Input: part model. Units: mm. Frame: model coordinates. A direction names the side the tool comes from. Round coordinates to 2 decimals unless told otherwise and drop trailing zeros. Loops run counter-clockwise (first coordinate to the right, second up) from the corner with the lowest first, then second, coordinate; pieces in that order, holes last. Notation, with made-up numbers: (28.5, 30.25) - (42.5, 30.25) arc R12 cw to (42.5, 34.25) - close; hole circle Ø3 at (7, 45). An arc over 180 degrees is marked (long way). Write each question's results on one line, items separated by ' | '.
Autodesk Inventor part; units mm, degrees
ref_plane "YZ Plane" through (0, 0, 0) normal (1, 0, 0) x (0, 1, 0)
ref_plane "XZ Plane" through (0, 0, 0) normal (0, 1, 0) x (-1, 0, 0)
ref_plane "XY Plane" through (0, 0, 0) normal (0, 0, 1) x (1, 0, 0)
sketch "Sketch1" plane through (0, 0, 0) normal (0, 1, 0) x (-1, 0, 0)
  line L0 (5, 0) -> (31, 0)
  line L1 (36, -30) -> (36, -120)
  line L2 (31, -150) -> (5, -150)
  line L3 (0, -120) -> (0, -30)
  circle A0 centre (18, -25) radius 5.1
  circle A1 centre (18, -55) radius 5.1
  circle A2 centre (18, -85) radius 5.1
  circle A3 centre (18, -125) radius 5.1
  line L4 (36, -30) -> (31, -30)
  line L5 (31, -30) -> (31, -40)
  line L6 (31, -40) -> (36, -40)
  line L7 (36, -120) -> (31, -120)
  line L8 (31, -120) -> (31, -110)
  line L9 (31, -110) -> (36, -110)
  line L10 (0, -30) -> (5, -30)
  line L11 (5, -30) -> (5, -40)
  line L12 (5, -40) -> (0, -40)
  line L13 (0, -120) -> (5, -120)
  line L14 (5, -120) -> (5, -110)
  line L15 (0, -110) -> (5, -110)
  circle A4 centre (18, -25) radius 2.25
  circle A5 centre (18, -55) radius 2.25
  circle A6 centre (18, -85) radius 2.25
  circle A7 centre (18, -125) radius 2.25
  line L16 (5, 0) -> (0, -30)
  line L17 (31, -150) -> (36, -120)
  line L18 (5, -150) -> (0, -120)
  line L19 (31, 0) -> (36, -30)
  line L20 (18, -100) -> (13, -105)
  line L21 (13, -105) -> (18, -110)
  line L22 (23, -105) -> (18, -110)
  line L23 (23, -105) -> (18, -100)
  line L24 (21, -114.95) -> (18, -117.95)
  line L25 (15, -114.95) -> (18, -117.95)
  line L26 (15, -114.95) -> (18, -111.95)
  line L27 (18, -111.95) -> (21, -114.95)
  line L28 (21, -95.05) -> (18, -98.05)
  line L29 (18, -98.05) -> (15, -95.05)
  line L30 (15, -95.05) -> (18, -92.05)
  line L31 (18, -92.05) -> (21, -95.05)
  line L32 (31, -150) -> (28, -150)
  line L33 (5, -150) -> (8, -150)
  line L34 (8, -148) -> (28, -148)
  line L35 (8, -148) -> (8, -144)
  line L36 (8, -144) -> (28, -144)
  line L37 (28, -144) -> (28, -148)
  line L38 (31, 0) -> (28, 0)
  line L39 (5, 0) -> (8, 0)
  line L40 (8, -2) -> (28, -2)
  line L41 (28, -2) -> (28, -6)
  line L42 (28, -6) -> (8, -6)
  line L43 (8, -6) -> (8, -2)
  line L44 (36, -75) -> (36, -83)
  line L45 (36, -75) -> (36, -67)
  line L46 (36, -67) -> (28, -75)
  line L47 (36, -83) -> (28, -75)
  line L48 (0, -75) -> (0, -83)
  line L49 (0, -75) -> (0, -67)
  line L50 (0, -67) -> (8, -75)
  line L51 (0, -83) -> (8, -75)
  point P0 (0, 0)
  point P1 (18, 0)
  point P2 (18, -150)
  dimension "d2" = 10.2
  dimension "d3" = 25
  dimension "d4" = 10.2
  dimension "d5" = 30
  dimension "d6" = 10.2
  dimension "d7" = 30
  dimension "d8" = 10.2
  dimension "d9" = 40
  dimension "d10" = 25
  dimension "d12" = 5
  dimension "d13" = 10
  dimension "d15" = 10
  dimension "d17" = 5
  dimension "d19" = 5
  dimension "d22" = 4.5
  dimension "d23" = 4.5
  dimension "d24" = 4.5
  dimension "d25" = 4.5
  dimension "d38" = 3
  dimension "d39" = 2
  dimension "d41" = 2
  dimension "d42" = 4
  dimension "d44" = 2
  dimension "d45" = 3
  dimension "d46" = 4
  dimension "d50" = 8
  dimension "d51" = 8
extrude "Extrusion1" add sketch "Sketch1" along normal blind 5 contours L0 L19 L4 L5 L6 L1 L46 L47 L9 L8 L7 L17 L2 L18 L13 L14 L15 L3 L51 L50 L12 L11 L10 L16
extrude "Extrusion2" add sketch "Sketch1" along normal blind 1 contours A0 | A1 | A2 | A3
sketch "Sketch2" plane through (0, 5, 0) normal (0, 1, 0) x (1, 0, 0)
  line L0 (-36, 120) -> (-31, 120)
  line L1 (-33.5, 120) -> (-33.5, 135)
  line L2 (-31, 150) -> (-36, 120)
  line L3 (-33.5, 120) -> (-35.9995, 120)
  line L4 (-35.9995, 120) -> (-33.5, 135)
  line L5 (-31, 30) -> (-36, 30)
  line L6 (-33.5, 30) -> (-33.5, 15)
  line L7 (-36, 30) -> (-31, 0)
  line L8 (-33.5, 15) -> (-36, 30)
  line L9 (-36, 30) -> (-33.5, 30)
  point P0 (0, 0)
  dimension "d52" = 15
extrude "Extrusion3" add sketch "Sketch2" along normal blind 20
sketch "Sketch3" plane through (-36, 0, -120) normal (0, 0, 1) x (1, 0, 0)
  line L0 (2.5, 5) -> (2.5, 25)
  line L1 (0, 0) -> (0, 5)
  line L2 (2.5, 25) -> (0, 25)
  line L3 (0, 25) -> (0, 5)
  line L4 (0, 5) -> (2.5, 5)
  line L5 (2.5, 5) -> (2.5, 25)
  point P0 (36, 0)
extrude "Extrusion4" add sketch "Sketch3" along normal blind 20
sketch "Sketch4" plane through (-31, 0, -30) normal (0, 0, -1) x (-1, 0, 0)
  line L0 (5, 0) -> (5, 25)
  line L1 (2.5, 5) -> (5, 5)
  line L2 (5, 5) -> (5, 25)
  line L3 (5, 25) -> (2.5, 25)
  line L4 (2.5, 25) -> (2.5, 5)
  point P0 (-31, 0)
extrude "Extrusion5" add sketch "Sketch4" along normal blind 20
sketch "Sketch5" plane through (-33.5, 5, -135) normal (1, 0, 0) x (0, 0, -1)
  line L0 (0, 20) -> (-35, 20)
  line L1 (0, 20) -> (0, 10)
  line L2 (0, 0) -> (0, 20)
  line L3 (-35, 0) -> (-35, 20)
  line L4 (-35, 10) -> (-35, 20)
  line L5 (-35, 20) -> (0, 20)
  line L6 (-85, 20) -> (-85, 0)
  line L7 (-120, 20) -> (-85, 20)
  line L8 (-85, 10) -> (-120, 10)
  line L9 (-120, 10) -> (-120, 20)
  line L10 (-120, 20) -> (-85, 20)
  line L11 (-85, 20) -> (-85, 10)
  line L12 (0, 10) -> (-35, 10)
  line L13 (-35, 10) -> (-35, 20)
  line L14 (-35, 20) -> (0, 20)
  line L15 (0, 20) -> (0, 10)
  line L16 (0, 0) -> (-35, 0)
  line L17 (-35, 0) -> (-35, 15)
  line L18 (-35, 15) -> (0, 15)
  line L19 (0, 15) -> (0, 0)
  line L20 (-35, 15) -> (0, 15)
  line L21 (0, 15) -> (0, 20)
  line L22 (0, 20) -> (-35, 20)
  line L23 (-35, 20) -> (-35, 15)
  line L24 (-85, 15) -> (-120, 15)
  line L25 (-120, 15) -> (-120, 20)
  line L26 (-120, 20) -> (-85, 20)
  line L27 (-85, 20) -> (-85, 15)
  point P0 (-135, -5)
extrude "Extrusion6" add sketch "Sketch5" along normal blind 20 contours L1 L18 L3 L0 | L6 L24 L9 L7
fillet "Fillet1" radius 2 4 edges at (-13.5, 25, -117.5) (-13.5, 25, -32.5) (-23.5, 25, -15) (-23.5, 25, -135)
sketch "Sketch6" plane through (0, 25, 0) normal (0, 1, 0) x (1, 0, 0)
  circle A0 centre (-18, 125) radius 2.25
  circle A1 centre (-18, 125) radius 2.25
  circle A2 centre (-18, 25) radius 2.25
  circle A3 centre (-18, 25) radius 2.25
  circle A4 centre (-18, 125) radius 2.5
  circle A5 centre (-18, 25) radius 2.5
  point P0 (0, 0)
  dimension "d62" = 5
  dimension "d63" = 5
extrude "Extrusion7" cut sketch "Sketch6" against normal blind 20 contours A0 | A2 | A4 | A5
properties part number "SideV1"
1. Section query D-D, the plane z = -102. Output: boundary loops of the cut face in (x, y), plus the area to 3 significant figures.
Answer:
outline: (-36, 0) - (-20, 0) - (-20, 5) - (-33.5, 5) - (-33.5, 20) - (-13.5, 20) - (-13.5, 23) arc R2 ccw to (-15.5, 25) - (-36, 25) - close; (-16, 0) - (0, 0) - (0, 5) - (-16, 5) - close | area: 309 mm^2
2. Contact query for flat-ended pins moving along their axis: pin 1 (1.5 mm diameter, centred on x = -19, y = 21.5, fed in from -Z); pin 2 (5.5 mm diameter, centred on y = 1.5, z = -116, fed in from +X); pin 3 (12 mm diameter, centred on y = 12.5, z = -18.5, fed in from -X). Output: stop coordinate, or through.
Answer:
pin 1: z = -135 | pin 2: x = -5 | pin 3: x = -35.08
3. Section query A-A, the plane y = 21.5. Output: boundary loops of the cut face in (x, z), plus the area to 3 significant figures.
Answer:
outline: (-36, -120) - (-33.5, -135) - (-13.5, -135) - (-13.5, -100) - (-36, -100) - close; (-36, -50) - (-13.5, -50) - (-13.5, -15) - (-33.5, -15) - (-36, -30) - close; hole circle Ø5 at (-18, -125); hole circle Ø5 at (-18, -25) | area: 1,500 mm^2
4. Set-up query: faces 1 (the flat face through (-16.48, 2.46, -93.57)), 2 (the cylindrical face through (-18.33, 22.54, -127.48)), 3 (the flat face through (-34, 2, -30)), 4 (the flat face through (-27.2, 20.2, -50)). Return all of +Z, -Z, +X, -X, +Y, -Y with unobstructed straight access to the full face (end or side cutting, diameter ignored); none if empty.
Answer:
face 1: +Y, -Y | face 2: +Y | face 3: -X, -Y | face 4: +X, -X, +Y
5. Section query C-C, the plane y = 6.75. Output: boundary loops of the cut face in (x, z), plus the area to 4 significant figures.
Answer:
outline: (-36, -120) - (-33.5, -135) - (-33.5, -100) - (-36, -100) - close; (-36, -50) - (-33.5, -50) - (-33.5, -15) - (-36, -30) - close | area: 137.5 mm^2
6. Section query B-B, the plane z = -55. Output: boundary loops of the cut face in (x, y), plus the area to 3 significant figures.
Answer:
outline: (-36, 0) - (-20.25, 0) - (-20.25, 1) - (-23.1, 1) - (-23.1, 5) - (-36, 5) - close; (-15.75, 0) - (0, 0) - (0, 5) - (-12.9, 5) - (-12.9, 1) - (-15.75, 1) - close | area: 135 mm^2
7. Mould query, pull axis Z, two halves, no side actions, for faces 5 (the flat face through (-2.535, 2.465, -135.21)), 6 (the flat face through (-36, 13, -106)), 7 (the flat face through (-19.48, 2.46, -113.43)). Classes: pulls with the +Z half, pulls with the -Z half, needs draft (parallel to the pull), parting line crosses it, or undercut.
Answer:
face 5: pulls with the -Z half | face 6: needs draft | face 7: undercut
8. Line query: line 1 (Z direction, x = -17, y = 21.75); line 2 (Z direction, x = -31, y = 23); line 3 (Y direction, x = -21, z = -24.5). Output: solid intervals per line, ascending. Write a range as [from, to].
Answer:
line 1: [-135, -127.29], [-122.71, -100], [-50, -27.29], [-22.71, -15] | line 2: [-135, -100], [-50, -15] | line 3: [0, 1], [20, 25]
